Part print with two shaded views. Sizes in mm from the minimum x, y, z corner. A direction names the side the tool comes from. Coordinates: 2 decimals unless noted, no trailing zeros. Order: outer loops, then holes, each group sorted by start corner. A loop starts at its lowest first (then second) coordinate and runs counter-clockwise, first axis right, second up. Notation, with made-up numbers: (-31.5, 13) - (-5.5, 13) arc R25 ccw to (-5.5, 29) - close; hole circle Ø1 at (0, -25.75). An arc over 180 degrees is marked (long way). Write each question's results on one line, items separated by ' | '. Start each with the question number.
Q1. Band-saw the part on A-A, the plane y = 12. Write the cut outline in (x, z), then the cut area to 3 significant figures.
Q2. Pin check, flat tips, straight feed: P1, Ø2, axis at y = 20.5, z = 15, coming from the -X side; P2, Ø9, axis at x = 55, y = 12.5, coming from the +Z side. Stop position of each tip, or through.
Q3. Which spindle directions (+Z, -Z, +X, -X, +Y, -Y) get a long thin tool onto all of the face, cutting with end or side? Do the marked faces 5 and 6. Say none if no direction does.
Q4. Band-saw the part on B-B, the plane z = 16.5. Write the cut outline in (x, y).
Q5. Pull direction X, two halves, no side cores. Call the marked faces 1, 2, 3 and 4: released by +X, released by -X, zero draft, split by the parting line, or undercut.
Q6. Wall check: probe 1 along X at (y, z) = (17.5, 11.75); probe 2 along Z at (x, y) = (95, 27.5); probe 3 along X at (y, z) = (11, 17.25). Give the ranges that are in metal, low to high.
Q7. Band-saw the part on D-D, the plane y = 19. Write the cut outline in (x, z).
Q8. Band-saw the part on C-C, the plane x = 40. Write the cut outline in (y, z).
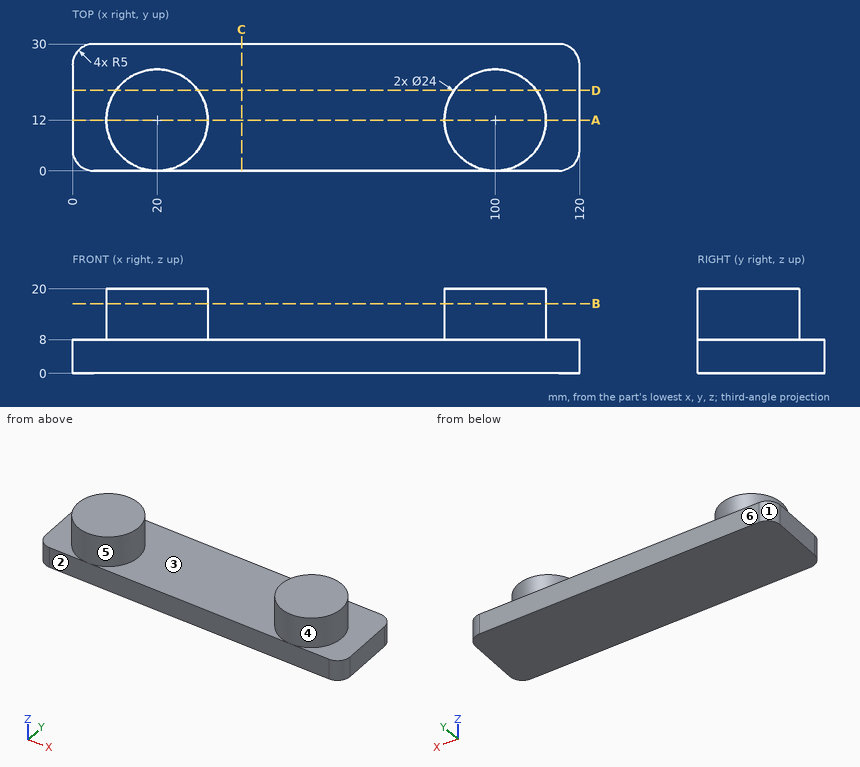
Results below:
1) outline: (0, 0) - (120, 0) - (120, 8) - (112, 8) - (112, 20) - (88, 20) - (88, 8) - (32, 8) - (32, 20) - (8, 20) - (8, 8) - (0, 8) - close | area: 1,540 mm²
2) P1: stops at x = 10.63 | P2: stops at z = 8
3) face 5: +Z | face 6: +Z, -Z, +X, -X, +Y
4) outline: circle Ø24 at (20, 12); circle Ø24 at (100, 12)
5) face 1: released by -X | face 2: zero draft | face 3: undercut | face 4: undercut
6) probe 1: x = 9.33 to 30.67, 89.33 to 110.67 | probe 2: z = 0 to 8 | probe 3: x = 8.04 to 31.96, 88.04 to 111.96
7) outline: (0, 0) - (120, 0) - (120, 8) - (109.75, 8) - (109.75, 20) - (90.25, 20) - (90.25, 8) - (29.75, 8) - (29.75, 20) - (10.25, 20) - (10.25, 8) - (0, 8) - close
8) outline: (0, 0) - (30, 0) - (30, 8) - (0, 8) - close
